Work out the finished part from the listing and answer in its coordinate system (mm). A direction names the side the tool comes from. Give positions to 0.01 mm unless a question says otherwise; leave off trailing zeros. Loops run counter-clockwise (first coordinate to the right, second up) from the corner with the lowest first, then second, coordinate; pieces in that order, holes last.
from build123d import *

# Parameters (mm, degrees)
CORTE_EXTRUS_O1_DEPTH = 4


with BuildPart() as part:
    # Esboço1 → Revolução1 (revolve)
    with BuildSketch(Plane.XY):
        with BuildLine():
            Line((0, 0), (2.5, 0))
            Line((2.5, 0), (2.5, 30))
            Line((2.5, 30), (4.75, 30))
            Line((4.75, 30), (4.75, 30.4))
            ThreePointArc((4.75, 30.4), (4.054378605, 32.079378605), (2.375, 32.775))
            Line((2.375, 32.775), (0, 32.775))
            Line((0, 32.775), (0, 0))
        make_face()
    revolve(axis=Axis((0, 32.775, 0), (0, -1, 0)))

    # Esboço2 → Corte-extrusão1 (cut)
    with BuildSketch(Plane(origin=(0, 32.775, 0), x_dir=(1, 0, 0), z_dir=(0, 1, 0))):
        Polygon((-1.5, 0.866025404), (-1.5, -0.866025404), (0, -1.732050808), (1.5, -0.866025404), (1.5, 0.866025404), (0, 1.732050808), align=None)
    extrude(amount=-CORTE_EXTRUS_O1_DEPTH, mode=Mode.SUBTRACT)


solid = part.part
Item 1: Find section A-A, the plane y = 8. Write down the section's boundary in (x, z).
Item 2: Flat-ended cylindrical pins translate along their axes: pin 1 Ø1.5 at (x, y) = (0.5, 20.5) entering from -Z; pin 2 Ø1 at (y, z) = (5, -1.5) entering from +X; pin 3 Ø4 at (y, z) = (20, 2.5) entering from +X. Find the tip coordinate at first contact, or state that the pin passes through.
Item 3: Determine the mould class of faces 4 (the face through (1.5, 31, 0)), 5 (the face through (2, 32.775, 0)), 6 (the face through (-0.76, 30.803, 1.293)), 7 (the face through (2.192, 30.203, -4.214)) for opening direction Z: released by +Z, released by -Z, zero draft, split by the parting line, or undercut.
Item 4: For faces 1 (the face through (0, 0, 0)), 2 (the face through (0, 28.775, 0)), 3 (the face through (-2, 30, -2)), determine the directions among +Z, -Z, +X, -X, +Y, -Y from which every point of the face is accessible in a straight line to the end or side of a thin tool.
Item 5: Consider line 1 (Z direction, x = -2, y = 29.5); line 2 (Y direction, x = -0.25, z = -0.75) (3 decimals). Determine where each line is inside the solid, lowest interval first.
Ans:
1. outline: circle Ø5 at (0, 0)
2. pin 1: stops at z = -2.5
2. pin 2: stops at x = 2.29
2. pin 3: stops at x = 2.45
3. face 4: undercut
3. face 5: zero draft
3. face 6: undercut
3. face 7: split by the parting line
4. face 1: +Z, -Z, +X, -X, -Y
4. face 2: +Y
4. face 3: -Y
5. line 1: z = -1.5 to 1.5
5. line 2: y = 0 to 28.775
